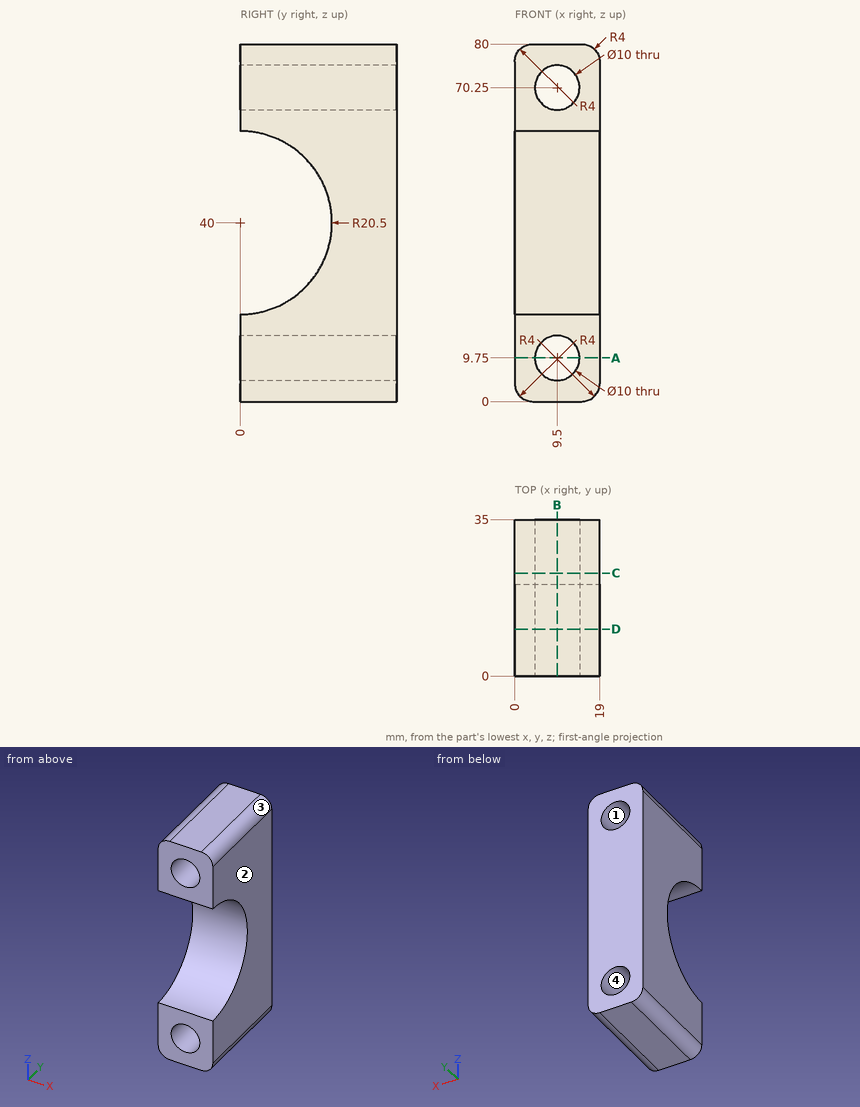
Can you work these out from the drawing? Everything is in mm from the part's minimum corner. Coordinates: 2 decimals unless noted, no trailing zeros. Loops run counter-clockwise (first coordinate to the right, second up) from the corner with the lowest first, then second, coordinate; pieces in that order, holes last. Notation, with made-up numbers: (-33, -8) - (-2, -8) arc R27 ccw to (-2, 11) - close; hole circle Ø3 at (48.25, -10). An arc over 180 degrees is marked (long way). Answer as CSV lines item,"result".
Q1. If we section it at D-D, the plane y = 10.5: Write out the boundary of the cut face in (x, z), and give its area (3 significant figures).
Response:
outline,"(0, 4) arc R4 ccw to (4, 0) - (15, 0) arc R4 ccw to (19, 4) - (19, 22.39) - (0, 22.39) - close; (0, 57.61) - (19, 57.61) - (19, 76) arc R4 ccw to (15, 80) - (4, 80) arc R4 ccw to (0, 76) - close; hole circle Ø10 at (9.5, 9.75); hole circle Ø10 at (9.5, 70.25)"
area,"680 mm2"
Q2. We'd pull the mould along Z, two halves only. Please class the marked faces 1, 2, 3 and 4: pulls with the +Z half, pulls with the -Z half, needs draft (parallel to the pull), parting line crosses it, or undercut.
Response:
face 1,"undercut"
face 2,"needs draft"
face 3,"pulls with the +Z half"
face 4,"undercut"
Q3. If we section it at C-C, the plane y = 23: Write out the boundary of the cut face in (x, z).
Response:
outline,"(0, 4) arc R4 ccw to (4, 0) - (15, 0) arc R4 ccw to (19, 4) - (19, 76) arc R4 ccw to (15, 80) - (4, 80) arc R4 ccw to (0, 76) - close; hole circle Ø10 at (9.5, 9.75); hole circle Ø10 at (9.5, 70.25)"
Q4. If we section it at A-A, the plane z = 9.75: Write out the boundary of the cut face in (x, y), and give its area (3 significant figures).
Response:
outline,"(0, 0) - (4.5, 0) - (4.5, 35) - (0, 35) - close; (14.5, 0) - (19, 0) - (19, 35) - (14.5, 35) - close"
area,"315 mm2"
Q5. If I drill on L1, parallel to X at y = 10.5, z = 70.25; L2, parallel to Z at x = 11.25, y = 13; L3, parallel to Z at x = 8, y = 26, over which ranges is the centre line in solid material (lowest first)? Write a range as [from, to].
Response:
L1,"[0, 4.5], [14.5, 19]"
L2,"[0, 5.07], [14.43, 24.15], [55.85, 65.57], [74.93, 80]"
L3,"[0, 4.98], [14.52, 65.48], [75.02, 80]"
Q6. For pin 1 (8 mm diameter, centred on x = 9.5, z = 70.25, fed in from +Y), with a flat end and sliding along its axis, tell me the tip position at first contact or that it passes through.
Response:
pin 1,"through"
Q7. If we section it at B-B, the plane x = 9.5: Write out the boundary of the cut face in (y, z), and give its area (3 significant figures).
Response:
outline,"(0, 0) - (35, 0) - (35, 4.75) - (0, 4.75) - close; (0, 14.75) - (35, 14.75) - (35, 65.25) - (0, 65.25) - (0, 60.5) arc R20.5 cw to (0, 19.5) - close; (0, 75.25) - (35, 75.25) - (35, 80) - (0, 80) - close"
area,"1,440 mm2"
